```python
from build123d import *

# Parameters (mm, degrees)
CHAMFER1_SIZE      = 1
CUT_EXTRUDE1_DEPTH = 3.5


with BuildPart() as part:
    # Sketch1 → Revolve1 (revolve)
    with BuildSketch(Plane.XY):
        Polygon((0, 0), (7.5, 0), (7.5, -9), (11, -9), (11, -39), (9, -39), (9, -56), (7.5, -56), (7.5, -65), (0, -65), align=None)
    revolve(axis=Axis((0, -65, 0), (0, 1, 0)))

    # Chamfer1
    chamfer1_edges = [part.edges().sort_by_distance(p)[0] for p in [
        (-7.5, 0, 0),
        (-7.5, -65, 0),
        (-9, -56, 0),
    ]]
    chamfer(chamfer1_edges, length=CHAMFER1_SIZE)

    # Sketch4 → Cut-Extrude1 (cut)
    with BuildSketch(Plane.XY.offset(9)):
        with BuildLine():
            Line((2.952489762, -42), (2.952489762, -50))
            ThreePointArc((2.952489762, -50), (0, -52.952489762), (-2.952489762, -50))
            Line((-2.952489762, -50), (-2.952489762, -42))
            ThreePointArc((-2.952489762, -42), (0, -39.047510238), (2.952489762, -42))
        make_face()
    extrude(amount=-CUT_EXTRUDE1_DEPTH, mode=Mode.SUBTRACT)


solid = part.part
```
The listing builds one solid part. Answer for the finished solid, in the listing's coordinates (mm). A direction names the side the tool comes from. Give positions to 0.01 mm unless a question says otherwise; leave off trailing zeros. Loops run counter-clockwise (first coordinate to the right, second up) from the corner with the lowest first, then second, coordinate; pieces in that order, holes last. Notation, with made-up numbers: M 36,87 L 43,87 A17 cw 43,113 Z; hole C 70.25,-39 d9. An arc over 180 degrees is marked long. One line per item, written item: value.
Q1. A cutting plane is placed at A-A on z = 0. Determine the outline of the cut face in (x, y).
Working result:
outline: M -11,-39 L -9,-39 L -9,-55 L -8,-56 L -7.5,-56 L -7.5,-64 L -6.5,-65 L 6.5,-65 L 7.5,-64 L 7.5,-56 L 8,-56 L 9,-55 L 9,-39 L 11,-39 L 11,-9 L 7.5,-9 L 7.5,-1 L 6.5,0 L -6.5,0 L -7.5,-1 L -7.5,-9 L -11,-9 Z
Q2. Find the intervals of material crossed by line 1 (Y direction, x = 9.5, z = 4); line 2 (Y direction, x = 1, z = 7.25); line 3 (X direction, y = -48, z = 0), in increasing order. Write a range as from..to.
Working result:
line 1: y = -39..-9
line 2: y = -64.18..-52.78, -39.22..-0.82
line 3: x = -9..9
Q3. Flat-ended cylindrical pins translate along their axes: P1, Ø3.5, axis at y = -47.5, z = 7.5, coming from the +X side; P2, Ø1.8, axis at x = 0.5, y = -43.5, coming from the +Z side; P3, Ø1.5, axis at x = -3.5, z = 8.5, coming from the -Y side. Find the tip coordinate at first contact, or state that the pin passes through.
Working result:
P1: stops at x = 6.92
P2: stops at z = 5.5
P3: stops at y = -55.56
Q4. A cutting plane is placed at B-B on x = 0. Determine the outline of the cut face in (y, z).
Working result:
outline: M -65,-6.5 L -64,-7.5 L -56,-7.5 L -56,-8 L -55,-9 L -39,-9 L -39,-11 L -9,-11 L -9,-7.5 L -1,-7.5 L 0,-6.5 L 0,6.5 L -1,7.5 L -9,7.5 L -9,11 L -39,11 L -39,9 L -39.05,9 L -39.05,5.5 L -52.95,5.5 L -52.95,9 L -55,9 L -56,8 L -56,7.5 L -64,7.5 L -65,6.5 Z
Q5. Determine the mould class of faces 5 (the face through (-2.952, -46, 7)), 6 (the face through (-7.493, -5.056, -0.33)), 7 (the face through (0.06, -52.95, 7.28)), 8 (the face through (0, 0, 0)) for opening direction Y: +Y half, -Y half, draft (parallel to the pull), parting line (faces both ways), or undercut.
Working result:
face 5: undercut
face 6: draft
face 7: undercut
face 8: +Y half
Q6. A cutting plane is placed at C-C on y = -27.5. Determine the outline of the cut face in (x, z), then the cut area to 3 significant figures.
Working result:
outline: C 0,0 d22
area: 380 mm^2
Q7. For faces 1 (the face through (-7.2, -9, -2.6)), 2 (the face through (-1.172, -47.112, -8.923)), 3 (the face through (2.952, -46, 7)), 4 (the face through (0, -65, 0)), determine the directions among +Z, -Z, +X, -X, +Y, -Y from which every point of the face is accessible in a straight line to the end or side of a thin tool.
Working result:
face 1: +Y
face 2: -Y
face 3: +Z
face 4: +Z, -Z, +X, -X, -Y
